The model under review builds one solid part; all positions refer to its coordinate system, in mm. A direction names the side the tool comes from. Coordinates: 2 decimals unless noted, no trailing zeros. Order: outer loops, then holes, each group sorted by start corner. A loop starts at its lowest first (then second) coordinate and runs counter-clockwise, first axis right, second up. Notation, with made-up numbers: M 65,42.5 L 73,42.5 A22 ccw 73,52.5 Z; hole C 16,28 d11. An arc over 180 degrees is marked long. Answer as CSV lines item,"result". Start each with the question number.
Q1. The part is to be moulded in two halves that separate along Z. For faces 4 (the face through (6, -4, 54.827)), 5 (the face through (9, -20, -170.173)), 6 (the face through (8.874, -39.398, -59.953)), 7 (the face through (9, -49.395, -119)), say which applies: +Z half, -Z half, draft (parallel to the pull), parting line (faces both ways), or undercut.
Q2. Consider section C-C on z = 43. Write out the cut boundary in (x, y), and give its area (3 significant figures).
Q3. Machinability: for faces 1 (the face through (15, -19, -15.173)), 2 (the face through (18, -19, -92)), 3 (the face through (6, -34, 54.827)), which of the approach directions +Z, -Z, +X, -X, +Y, -Y give a long, thin tool a straight path to every point of the face, cutting with its end or side? Answer none if there is none.
Q4. For P1, Ø2, axis at x = 7, y = -4, coming from the +Z side, flat-tipped, find the tip position at first contact; note if it passes through.
Q5. Consider section A-A on x = 6.25. Write out the cut boundary in (y, z), and give its area (3 significant figures).
Q6. Wall thickness on L1, parallel to Y at x = 6.25, z = 61.75; L2, parallel to X at y = -5.5, z = 26; L3, parallel to Z at x = 12, y = -36.5: over which ranges is each line inside the solid? List them lowest first. Write a range as [from, to].
Q7. Consider section B-B on y = -13.5. Write out the cut boundary in (x, z).
from build123d import *

# Parameters (mm, degrees)
ESQUISSE1_W             = 80
ESQUISSE1_H             = 60
ESQUISSE1_R             = 2
BOSS_EXTRU_2_DEPTH      = 12.5
ESQUISSE1_3_R           = 2
BOSS_EXTRU_3_DEPTH      = 18
ESQUISSE5_R             = 2
ENL_V_MAT_EXTRU_2_DEPTH = 10


with BuildPart() as part:
    # Esquisse1 → Boss.-Extru.2 (new body)
    with BuildSketch(Plane(origin=(0, 0, 0), x_dir=(0, 0, -1), z_dir=(1, 0, 0))):
        with Locations((-24.826777374, -19.395329297)):
            Rectangle(ESQUISSE1_W, ESQUISSE1_H)
        with Locations((-54.826777374, 5.154670703)):
            Circle(ESQUISSE1_R, mode=Mode.SUBTRACT)
        with Locations((5.173222626, 5.154670703)):
            Circle(ESQUISSE1_R, mode=Mode.SUBTRACT)
    extrude(amount=BOSS_EXTRU_2_DEPTH)

    # Esquisse1<3> → Boss.-Extru.3 (add)
    with BuildSketch(Plane(origin=(0, 0, 0), x_dir=(0, 0, -1), z_dir=(1, 0, 0))):
        with BuildLine():
            Line((170.173222626, 10.604670703), (15.173222626, 10.604670703))
            Line((15.173222626, 10.604670703), (15.173222626, -49.395329297))
            Line((15.173222626, -49.395329297), (50.173222626, -49.395329297))
            ThreePointArc((50.173222626, -49.395329297), (60.173222626, -39.395329297), (70.173222626, -49.395329297))
            Line((70.173222626, -49.395329297), (170.173222626, -49.395329297))
            Line((170.173222626, -49.395329297), (170.173222626, 10.604670703))
        make_face()
        with Locations((116.173222626, -35.395329297)):
            Circle(ESQUISSE1_3_R, mode=Mode.SUBTRACT)
        with Locations((147.173222626, -35.395329297)):
            Circle(ESQUISSE1_3_R, mode=Mode.SUBTRACT)
    extrude(amount=BOSS_EXTRU_3_DEPTH)

    # Esquisse5 → Enlèv. mat.-Extru.2 (cut)
    with BuildSketch(Plane.XY.offset(64.826777374)):
        with Locations((6.25, -4.395329297)):
            Circle(ESQUISSE5_R)
        with Locations((6.25, -34.395329297)):
            Circle(ESQUISSE5_R)
    extrude(amount=-ENL_V_MAT_EXTRU_2_DEPTH, mode=Mode.SUBTRACT)


solid = part.part
Evaluation:
1,face 4,"+Z half"
1,face 5,"-Z half"
1,face 6,"undercut"
1,face 7,"draft"
2,outline,"M 0,-49.4 L 12.5,-49.4 L 12.5,10.6 L 0,10.6 Z"
2,area,"750 mm²"
3,face 1,"+Z, +X, +Y, -Y"
3,face 2,"+Z, -Z, +X, +Y, -Y"
3,face 3,"+Z"
4,P1,"stops at z = 54.83"
5,outline,"M -49.4,-170.17 L 10.6,-170.17 L 10.6,64.83 L -2.4,64.83 L -2.4,54.83 L -6.4,54.83 L -6.4,64.83 L -32.4,64.83 L -32.4,54.83 L -36.4,54.83 L -36.4,64.83 L -49.4,64.83 L -49.4,-50.17 A10 cw -49.4,-70.17 Z; hole C -35.4,-147.17 d4; hole C -35.4,-116.17 d4; hole C 5.15,-5.17 d4; hole C 5.15,54.83 d4"
5,area,"13,800 mm²"
6,L1,"y = [-49.4, -36.4], [-32.4, -6.4], [-2.4, 10.6]"
6,L2,"x = [0, 12.5]"
6,L3,"z = [-170.17, -148.84], [-145.51, -117.84], [-114.51, 64.83]"
7,outline,"M 0,-170.17 L 18,-170.17 L 18,-15.17 L 12.5,-15.17 L 12.5,64.83 L 0,64.83 Z"
